Here's how the part is built. I have some questions about the finished solid (model axes, mm). Coordinates: 2 decimals unless noted, no trailing zeros. Write each loop counter-clockwise with the first axis right and the second up, starting at its lowest first coordinate (ties: lowest second). Pieces come first, ordered by that corner, then holes. Notation, with made-up numbers: M -23,-2.75 L 9,-2.75 A23 cw 9,19.25 Z; hole C 52.25,-17.5 d4. An arc over 180 degrees is marked long. Use a Markdown table: item, result.
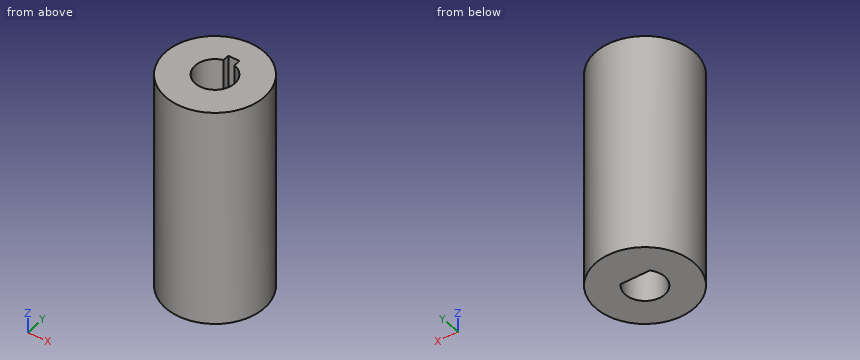
```python
from build123d import *

# Parameters (mm, degrees)
F0_R     = 11.1125
F0_R_2   = 4.445
F1_DEPTH = 25.4
F2_R     = 11.1125
F3_DEPTH = 11.43
F4_R     = 11.1125
F5_DEPTH = 12.7


with BuildPart() as f1:
    # F0 (on Top) → F1 (new body)
    with BuildSketch(Plane.XY):
        Circle(F0_R)
        Circle(F0_R_2, mode=Mode.SUBTRACT)
    extrude(amount=F1_DEPTH)

    # F2 (on face) → F3 (join)
    with BuildSketch(Plane(origin=(0, 0, 0), x_dir=(1, 0, 0), z_dir=(0, 0, -1))):
        Circle(F2_R)
        with BuildLine():
            ThreePointArc((-3.302, -2.975705), (0, 4.445), (3.302, -2.975705))
            Line((3.302, -2.975705), (-3.302, -2.975705))
        make_face(mode=Mode.SUBTRACT)
    extrude(amount=F3_DEPTH)

    # F4 (on face) → F5 (join)
    with BuildSketch(Plane.XY.offset(25.4)):
        Circle(F4_R)
        with BuildLine():
            ThreePointArc((4.445, 0), (-2.656396, -3.563929), (-1.27, 4.259709))
            Line((-1.27, 4.259709), (-1.27, 5.783709))
            Line((-1.27, 5.783709), (1.27, 5.783709))
            Line((1.27, 5.783709), (1.27, 4.259709))
            ThreePointArc((1.27, 4.259709), (3.563929, 2.656396), (4.445, 0))
        make_face(mode=Mode.SUBTRACT)
    extrude(amount=F5_DEPTH)


solid = f1.part
```
1. Suppose I cut it at A-A on x = 0. Write out the boundary of the cut face in (y, z) (1 decimal).
Answers follow:
| item | result |
|---|---|
| outline | M -11.1,-11.4 L -4.4,-11.4 L -4.4,38.1 L -11.1,38.1 Z; M 3,-11.4 L 11.1,-11.4 L 11.1,38.1 L 5.8,38.1 L 5.8,25.4 L 4.4,25.4 L 4.4,0 L 3,0 Z |
2. Suppose I cut it at C-C on z = 16.5. Write out the boundary of the cut face in (x, y) (1 decimal).
Answers follow:
| item | result |
|---|---|
| outline | C 0,0 d22.2; hole C 0,0 d8.9 |
3. Will these pins go through, and if not, where does the flat tip stop? pin 1 Ø1 at (x, z) = (-4, 2) entering from +Y; pin 2 Ø1.6 at (x, y) = (-0.5, 3.5) entering from +Z; pin 3 Ø5.5 at (x, y) = (0, 0) entering from -Z; pin 4 Ø1.7 at (y, z) = (5.5, 34) entering from +X.
Answers follow:
| item | result |
|---|---|
| pin 1 | stops at y = 10.55 |
| pin 2 | stops at z = 0 |
| pin 3 | passes through |
| pin 4 | stops at x = 10.09 |
4. I need wall thicknesses on probe 1 along X at (y, z) = (0, 11.5) (1 decimal); probe 2 along Z at (x, y) = (-1.75, 3.25). Which ranges of each line are inside material? Lowest first, please.
Answers follow:
| item | result |
|---|---|
| probe 1 | x = -11.1 to -4.4, 4.4 to 11.1 |
| probe 2 | z = -11.43 to 0 |
5. Suppose I cut it at B-B on y = 0.5. Write out the boundary of the cut face in (x, z).
Answers follow:
| item | result |
|---|---|
| outline | M -11.1,-11.43 L -4.42,-11.43 L -4.42,38.1 L -11.1,38.1 Z; M 4.42,-11.43 L 11.1,-11.43 L 11.1,38.1 L 4.42,38.1 Z |
6. Suppose I cut it at D-D on y = 8.5. Write out the boundary of the cut face in (x, z), and give its area (3 significant figures).
Answers follow:
| item | result |
|---|---|
| outline | M -7.16,-11.43 L 7.16,-11.43 L 7.16,38.1 L -7.16,38.1 Z |
| area | 709 mm2 |
